Source: CAD feature listing. Evaluate the final solid. Frame: model axes, mm. Face numbers are marked on the shaded views. A direction names the side the tool comes from. Coordinates: 2 decimals unless noted, no trailing zeros. Order: outer loops, then holes, each group sorted by start corner. A loop starts at its lowest first (then second) coordinate and runs counter-clockwise, first axis right, second up.
Item 1: Contact query for flat-ended pins moving along their axis: P1, Ø8, axis at x = 1.5, z = -10.5, coming from the -Y side; P2, Ø1.8, axis at y = 6, z = -1, coming from the -X side. Output: stop coordinate, or through.
Item 2: Section C-C on z = 5. Return the cut outline in (x, y), then the cut area to 3 significant figures.
Item 3: Mould query, pull axis Z, two halves, no side actions, for the marked faces 4, 5, 6 and 7. Classes: released by +Z, released by -Z, zero draft, split by the parting line, or undercut.
Item 4: Section B-B on x = -4.5. Return the cut outline in (y, z).
Item 5: Ray query, line 1 (Z direction, x = 0, y = 5.25); line 2 (X direction, y = 4, z = -12); line 3 (X direction, y = 5.5, z = 4). Return the intervals inside material, ascending.
Item 6: Reachability of the marked faces 1, 2 and 3 from +Z, -Z, +X, -X, +Y, -Y: full face, straight path, thin tool, end or side. Return the list, or none.
Item 7: Section A-A on z = 15. Return the cut outline in (x, y).
Item 8: Section D-D on y = 2.5. Return the cut outline in (x, z) (3 decimals).
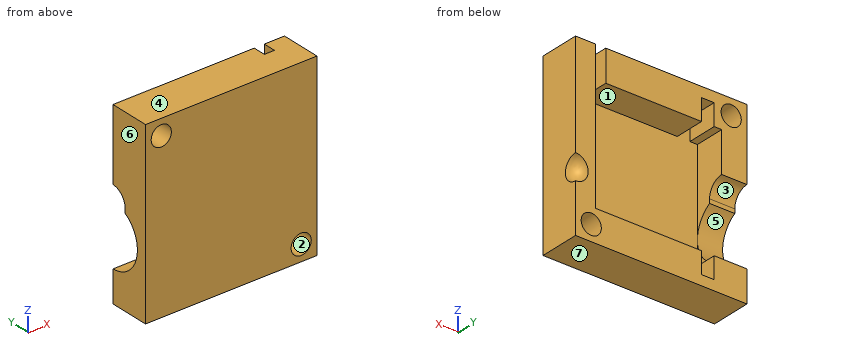
Autodesk Inventor part; units mm, degrees
ref_plane "YZ Plane" through (0, 0, 0) normal (1, 0, 0) x (0, 1, 0)
ref_plane "XZ Plane" through (0, 0, 0) normal (0, 1, 0) x (-1, 0, 0)
ref_plane "XY Plane" through (0, 0, 0) normal (0, 0, 1) x (1, 0, 0)
sketch "Sketch1" plane through (0, 0, 0) normal (0, 1, 0) x (-1, 0, 0)
  line L0 (16, 17.75) -> (-16, 17.75)
  line L1 (-16, 17.75) -> (-16, -17.75)
  line L2 (-16, -17.75) -> (16, -17.75)
  line L3 (16, -17.75) -> (16, 17.75)
  line L4 (16, 17.75) -> (-16, -17.75) construction
  line L5 (-16, 17.75) -> (16, -17.75) construction
  point P0 (0, 0)
  dimension "d0" = 32
  dimension "d1" = 35.5
extrude "Extrusion1" add sketch "Sketch1" along normal blind 8
sketch "Sketch2" plane through (0, 8, 0) normal (0, 1, 0) x (1, 0, 0)
  line L0 (-11, 11.5) -> (14, 11.5)
  line L1 (14, 11.5) -> (14, -11.5)
  line L2 (14, -11.5) -> (-11, -11.5)
  line L3 (-11, -11.5) -> (-11, 11.5)
  line L4 (-11, 11.5) -> (14, -11.5) construction
  line L5 (14, 11.5) -> (-11, -11.5) construction
  line L6 (16, -17.75) -> (16, 17.75)
  point P0 (0, 0)
  point P1 (1.5, 0)
  dimension "d4" = 0
  dimension "d5" = 2
  dimension "d6" = 25
  dimension "d13" = 23
extrude "Extrusion2" cut sketch "Sketch2" against normal blind 6
sketch "Sketch3" plane through (0, 8, 0) normal (0, 1, 0) x (1, 0, 0)
  line L0 (-7, -15.75) -> (-9.5, -15.75)
  line L1 (-9.5, -15.75) -> (-9.5, 15.75)
  line L2 (-9.5, 15.75) -> (-7, 15.75)
  line L3 (-7, 15.75) -> (-7, -15.75)
  line L4 (-7, -15.75) -> (-9.5, 15.75) construction
  line L5 (-9.5, -15.75) -> (-7, 15.75) construction
  line L6 (14, 11.5) -> (14, -11.5)
  point P0 (0, 0)
  point P1 (-8.25, 0)
  dimension "d9" = 21
  dimension "d10" = 2.5
  dimension "d11" = 0
  dimension "d12" = 31.5
extrude "Extrusion3" cut sketch "Sketch3" against normal blind 6
sketch "Sketch4" plane through (-16, 0, -17.75) normal (-1, 0, 0) x (0, 0, 1)
  line L0 (6.25, 8) -> (6.25, 2)
  line L1 (6.25, 8) -> (29.25, 8)
  line L2 (6.25, 2) -> (29.25, 2)
  line L3 (18.25, 5) -> (17.4462, 5)
  line L4 (18.25, 11) -> (17.4462, 11)
  arc A0 (18.25, 5) -> (18.25, 11) centre (18.25, 8) ccw
  arc A1 (17.4462, 11) -> (17.4462, 5) centre (12.25, 8) ccw
  arc A2 (18.25, 8) -> (17.5, 10.9047) centre (12.25, 8) ccw
  point P0 (17.75, 0)
  dimension "d17" = 6
extrude "Extrusion4" cut sketch "Sketch4" against normal up to surface (30 mm away) contours A1 L4 A0 L1 | L1 A0 L3 A1
thicken "Thicken1" operation add thickness 2 both sides no extend neighbours yes toward (1, 0, 0) faces at (16, 5.3333, 5.9167)
sketch "Sketch6" plane through (18, 0, 17.75) normal (1, 0, 0) x (0, 0, -1)
  arc A0 (18.0538, 5) -> (29.25, 8) centre (23.25, 8) ccw
  circle A1 centre (23.25, 8) radius 2.5
  point P0 (17.75, 0)
  dimension "d26" = 5
extrude "Extrusion6" cut sketch "Sketch6" against normal blind 2.5
fillet "Fillet2" radius 2.5 1 edges at (15.5, 5.5, -5.5)
sketch "Sketch7" plane through (0, 8, 0) normal (0, 1, 0) x (1, 0, 0)
  arc A0 (18, 8) -> (18, 3) centre (18, 5.5) ccw
  line L0 (18, 8) -> (18, 17.75)
  line L1 (18, 17.75) -> (-16, 17.75)
  line L2 (-16, 17.75) -> (-16, 11.5)
  line L3 (-16, 11.5) -> (-11, 11.5)
  line L4 (-11, 11.5) -> (-9.5, 11.5)
  line L5 (-9.5, 11.5) -> (-9.5, 15.75)
  line L6 (-9.5, 15.75) -> (-7, 15.75)
  line L7 (-7, 15.75) -> (-7, 11.5)
  line L8 (-7, 11.5) -> (14, 11.5)
  line L9 (14, 11.5) -> (14, -11.5)
  line L10 (14, -11.5) -> (-7, -11.5)
  line L11 (-7, -11.5) -> (-7, -15.75)
  line L12 (-7, -15.75) -> (-9.5, -15.75)
  line L13 (-9.5, -15.75) -> (-9.5, -11.5)
  line L14 (-9.5, -11.5) -> (-11, -11.5)
  line L15 (-11, -11.5) -> (-11, -3.5)
  line L16 (-11, -3.5) -> (-16, -3.5)
  line L17 (-16, -3.5) -> (-16, -17.75)
  line L18 (-16, -17.75) -> (18, -17.75)
  line L19 (18, -17.75) -> (18, 3)
  line L20 (-16, -17.75) -> (18, -17.75)
  line L21 (14, -11.5) -> (12, -11.5)
  line L22 (12, -11.5) -> (12, -17.75)
  line L23 (12, -17.75) -> (14, -17.75)
  line L24 (14, -17.75) -> (14, -11.5)
  point P0 (0, 0)
  dimension "d30" = 2
extrude "Extrusion7" cut sketch "Sketch7" against normal blind 2.5 contours L18 L22 L10 L24
sketch "Sketch8" plane through (0, 8, 0) normal (0, 1, 0) x (1, 0, 0)
  line L0 (18, 17.75) -> (-16, 17.75)
  line L1 (18, 8) -> (18, 17.75)
  line L2 (-16, -17.75) -> (12, -17.75)
  line L3 (-16, -3.5) -> (-16, -17.75)
  point P0 (0, 0)
  point P1 (14.875, 14.625)
  point P2 (-12.875, -14.625)
  dimension "d33" = 3.125
  dimension "d34" = 3.125
  dimension "d35" = 3.125
  dimension "d36" = 3.125
hole "Hole1" at (14.875, 8, -14.625) at (-12.875, 8, 14.625) direction (0, -1, 0) diameter 4 end through all
properties part number "knee_motor_hemi"
Answer list:
1. P1: stops at y = 0
1. P2: stops at x = 14
2. outline: (-16, 0) - (18, 0) - (18, 8) - (14, 8) - (14, 2) - (-11, 2) - (-11, 8) - (-16, 8) - close
2. area: 122 mm2
3. face 4: released by +Z
3. face 5: undercut
3. face 6: zero draft
3. face 7: released by -Z
4. outline: (0, -17.75) - (8, -17.75) - (8, -11.5) - (2, -11.5) - (2, 11.5) - (8, 11.5) - (8, 17.75) - (0, 17.75) - close
5. line 1: z = -17.75 to -11.5, 11.5 to 17.75
5. line 2: x = -16 to -9.5, -7 to 18
5. line 3: x = -16 to -11, 14 to 18
6. face 1: +Y
6. face 2: +Y, -Y
6. face 3: -X, +Y
7. outline: (-16, 0) - (-14.84, 0) - (-14.84, 8) - (-16, 8) - close; (-10.91, 0) - (18, 0) - (18, 8) - (14, 8) - (14, 5.5) - (12, 5.5) - (12, 8) - (-7, 8) - (-7, 2) - (-9.5, 2) - (-9.5, 8) - (-10.91, 8) - close
8. outline: (-16, -17.75) - (18, -17.75) - (18, 17.75) - (-16, 17.75) - (-16, -3.102) - (-11, -3.102) - (-11, 11.5) - (-9.5, 11.5) - (-9.5, 15.75) - (-7, 15.75) - (-7, 11.5) - (14, 11.5) - (14, -11.5) - (-7, -11.5) - (-7, -15.75) - (-9.5, -15.75) - (-9.5, -11.5) - (-11, -11.5) - (-11, -7.898) - (-16, -7.898) - close; hole circle Ø4 at (-12.875, 14.625); hole circle Ø4 at (14.875, -14.625)
